```python
from build123d import *

# Parameters (mm, degrees)
EXTRUDE1_DEPTH      = 2.89052
EXTRUDE1_DEPTH_BACK = 0.508
SKETCH5_R           = 10.16
EXTRUDE2_DEPTH      = 6.35
CUT_EXTRUDE1_START  = -0.508
SKETCH3_R           = 3.175
CUT_EXTRUDE1_DEPTH  = 9.74852
SPLIT1_START        = -6.477
SPLIT1_OUTLINE_W    = 4.7625
SPLIT1_OUTLINE_H    = 9.779
SPLIT1_DEPTH        = 12.954


# Read off the part's stored shape, not the designer's step: Split1
with BuildPart() as part:
    # Sketch1 → Extrude1 (new, two sides: drawn at the far end of the back side and taken through both)
    with BuildSketch(Plane(origin=(0, 0, 0), x_dir=(1, 0, 0), z_dir=(0, 1, 0)).offset(-EXTRUDE1_DEPTH_BACK)):
        with BuildLine():
            ThreePointArc((-3.364632139, 23.11648266), (-8.939508898, 21.581883622), (-13.966667445, 18.724975848))
            ThreePointArc((-13.966667445, 18.724975848), (-14.132678071, 14.132678071), (-18.724975848, 13.966667445))
            ThreePointArc((-18.724975848, 13.966667445), (-21.581883622, 8.939508898), (-23.11648266, 3.364632139))
            ThreePointArc((-23.11648266, 3.364632139), (-19.986625, 0), (-23.11648266, -3.364632139))
            ThreePointArc((-23.11648266, -3.364632139), (-21.581883622, -8.939508898), (-18.724975848, -13.966667445))
            ThreePointArc((-18.724975848, -13.966667445), (-14.132678071, -14.132678071), (-13.966667445, -18.724975848))
            ThreePointArc((-13.966667445, -18.724975848), (-8.939508898, -21.581883622), (-3.364632139, -23.11648266))
            ThreePointArc((-3.364632139, -23.11648266), (0, -19.986625), (3.364632139, -23.11648266))
            ThreePointArc((3.364632139, -23.11648266), (8.939508898, -21.581883622), (13.966667445, -18.724975848))
            ThreePointArc((13.966667445, -18.724975848), (14.132678071, -14.132678071), (18.724975848, -13.966667445))
            ThreePointArc((18.724975848, -13.966667445), (21.581883622, -8.939508898), (23.11648266, -3.364632139))
            ThreePointArc((23.11648266, -3.364632139), (19.986625, 0), (23.11648266, 3.364632139))
            ThreePointArc((23.11648266, 3.364632139), (21.581883622, 8.939508898), (18.724975848, 13.966667445))
            ThreePointArc((18.724975848, 13.966667445), (14.132678071, 14.132678071), (13.966667445, 18.724975848))
            ThreePointArc((13.966667445, 18.724975848), (8.939508898, 21.581883622), (3.364632139, 23.11648266))
            ThreePointArc((3.364632139, 23.11648266), (0, 19.986625), (-3.364632139, 23.11648266))
        make_face()
    extrude(amount=EXTRUDE1_DEPTH + EXTRUDE1_DEPTH_BACK)

    # Sketch5 → Extrude2 (add)
    with BuildSketch(Plane(origin=(0, 2.89052, 0), x_dir=(-1, 0, 0), z_dir=(0, 1, 0))):
        with Locations(Location((0, 0, 0), (0, 0, 90))):
            Circle(SKETCH5_R)
    extrude(amount=EXTRUDE2_DEPTH)

    # Sketch3 → Cut-Extrude1 (cut)
    with BuildSketch(Plane(origin=(0, 0, 0), x_dir=(1, 0, 0), z_dir=(0, 1, 0)).offset(CUT_EXTRUDE1_START)):
        with Locations(Location((0, 0, 0), (0, 0, 270))):
            Circle(SKETCH3_R)
    extrude(amount=CUT_EXTRUDE1_DEPTH, mode=Mode.SUBTRACT)

    # Split1 outline → Split1 (cut)
    with BuildSketch(Plane.YZ.offset(SPLIT1_START)):
        with Locations((6.85927, 0)):
            Rectangle(SPLIT1_OUTLINE_W, SPLIT1_OUTLINE_H)
    extrude(amount=SPLIT1_DEPTH, mode=Mode.SUBTRACT)


solid = part.part
```
Could you check a few things on this model? Use its own coordinates, in mm. A direction names the side the tool comes from. Give positions to 0.01 mm unless a question says otherwise; leave off trailing zeros. Write each loop counter-clockwise with the first axis right and the second up, starting at its lowest first coordinate (ties: lowest second). Pieces come first, ordered by that corner, then holes. Notation, with made-up numbers: (57.25, -9.75) - (88.25, -9.75) arc R16 ccw to (88.25, 18.25) - close; hole circle Ø2 at (-33, 73.5). An arc over 180 degrees is marked (long way). One line per item, written item: value. Start each with the question number.
Item 1: If we mould it in two halves opening along X, with no side actions, what happens to faces 3 (the face through (0, 7, 4.89)), 4 (the face through (10.074, 6.021, -1.323)), 5 (the face through (5, -0.508, 0)), 6 (the face through (-21.551, 1.167, -9.014))? For each: +X half, -X half, draft (parallel to the pull), parting line (faces both ways), or undercut.
Item 2: Imagine slicing it at A-A, the plane x = 0. List the corners of the cut face in (y, z) for me (1 decimal), and give its area (3 significant figures).
Item 3: Which directions (+Z, -Z, +X, -X, +Y, -Y) give clear straight access to the entire face, cutting with the end or side of a thin tool? Please do faces 1 (the face through (-0.071, 1.167, 19.987)), 2 (the face through (-6.477, 7, 0)).
Item 4: Imagine slicing it at B-B, the plane z = 0. List the corners of the cut face in (x, y) for me (3 decimals), and give its area (3 significant figures).
Item 5: I'm going to push flat-ended pins straight in: pin 1 (1.4 mm diameter, centred on x = -3, y = 6, fed in from +Z); pin 2 (2 mm diameter, centred on x = 9.5, y = 7, fed in from +Z); pin 3 (4 mm diameter, centred on y = 7.5, z = 1, fed in from -X). Where does each tip first touch, or does it pass through?
Item 6: Imagine slicing it at C-C, the plane y = 7.75. List the corners of the cut face in (x, z) for me, and give its area (3 significant figures).
Item 7: Please list where these lines run through material, in increasing order: line 1 (Z direction, x = -0.5, y = 8.5); line 2 (Y direction, x = -10, z = 9.5); line 3 (X direction, y = 2.25, z = -2.5). Write a range as from..to.
Item 8: Imagine slicing it at D-D, the plane z = 8.5. List the corners of the cut face in (x, y) for me, and give its area (3 significant figures).
Geometry says:
1. face 3: undercut
1. face 4: parting line
1. face 5: draft
1. face 6: -X half
2. outline: (-0.5, -20) - (2.9, -20) - (2.9, -10.2) - (9.2, -10.2) - (9.2, -4.9) - (4.5, -4.9) - (4.5, -3.2) - (-0.5, -3.2) - close; (-0.5, 3.2) - (4.5, 3.2) - (4.5, 4.9) - (9.2, 4.9) - (9.2, 10.2) - (2.9, 10.2) - (2.9, 20) - (-0.5, 20) - close
2. area: 187 mm^2
3. face 1: +Z, +Y, -Y
3. face 2: +Y
4. outline: (-19.987, -0.508) - (-3.175, -0.508) - (-3.175, 4.478) - (-6.477, 4.478) - (-6.477, 9.241) - (-10.16, 9.241) - (-10.16, 2.891) - (-19.987, 2.891) - close; (3.175, -0.508) - (19.987, -0.508) - (19.987, 2.891) - (10.16, 2.891) - (10.16, 9.241) - (6.477, 9.241) - (6.477, 4.478) - (3.175, 4.478) - close
4. area: 172 mm^2
5. pin 1: z = 9.9
5. pin 2: z = 5.57
5. pin 3: x = -10.16
6. outline: circle Ø20.32 at (0, 0); hole (-6.48, -4.89) - (6.48, -4.89) - (6.48, 4.89) - (-6.48, 4.89) - close
6. area: 198 mm^2
7. line 1: -10.15..-4.89, 4.89..10.15
7. line 2: -0.51..2.89
7. line 3: -21.1..-1.96, 1.96..21.1
8. outline: (-21.76, -0.51) - (21.76, -0.51) - (21.76, 2.89) - (5.57, 2.89) - (5.57, 9.24) - (-5.57, 9.24) - (-5.57, 2.89) - (-21.76, 2.89) - close
8. area: 219 mm^2
